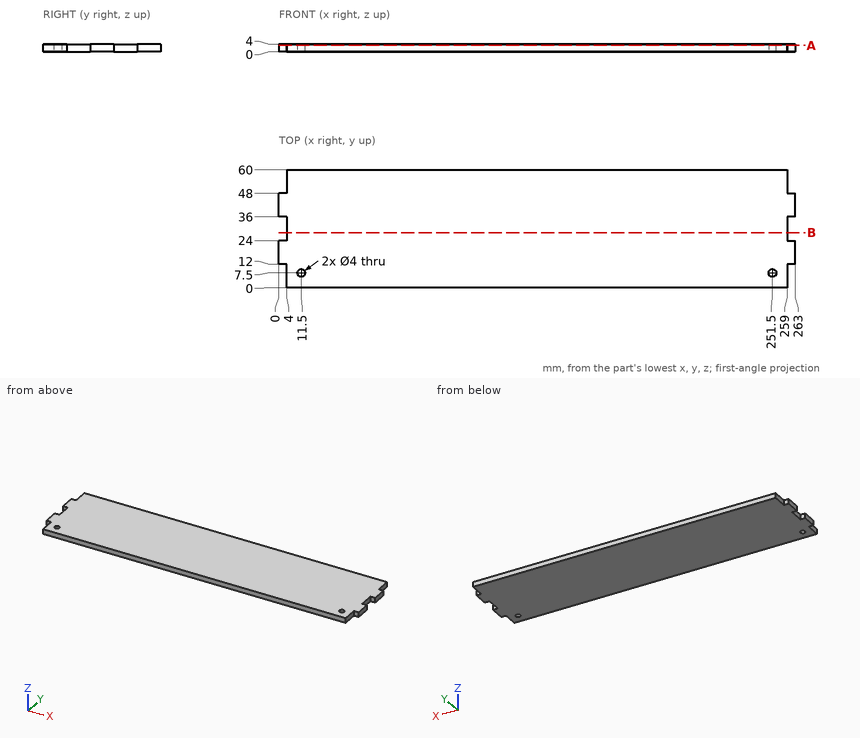
Study the drawing (mm; zero at the part's minimum x, y, z) and answer. Round coordinates to 2 decimals unless told otherwise and drop trailing zeros. Loops run counter-clockwise (first coordinate to the right, second up) from the corner with the lowest first, then second, coordinate; pieces in that order, holes last. Notation, with made-up numbers: (-1.5, 47.25) -> (7.5, 47.25) arc R18 ccw to (7.5, 59.25) -> close; hole circle Ø4 at (-26.5, 55.25). An arc over 180 degrees is marked (long way). One line per item, written item: value.
1) A cutting plane is placed at B-B (y = 28). Determine the outline of the cut face in (x, z), and give its area (3 significant figures).
Answer list:
outline: (4, 0) -> (259, 0) -> (259, 4) -> (4, 4) -> close
area: 1,020 mm²
2) Flat-ended cylindrical pins translate along their axes: P1, Ø1.2, axis at x = 2, z = 1, coming from the -Y side; P2, Ø1.2, axis at x = 2, z = 1, coming from the +Y side; P3, Ø1.2, axis at y = 31.5, z = 2, coming from the -X side. Find the tip coordinate at first contact, or state that the pin passes through.
Answer list:
P1: stops at y = 12
P2: stops at y = 48
P3: stops at x = 4
3) Consider L1, parallel to X at y = 7.5, z = 1.95; L2, parallel to Y at x = 251.5, z = 2.1; L3, parallel to X at y = 54.5, z = 2.5. Determine where each line is inside the solid, lowest interval first. Write a range as [from, to].
Answer list:
L1: x = [4, 9.5], [13.5, 249.5], [253.5, 259]
L2: y = [0, 5.5], [9.5, 60]
L3: x = [4, 259]
4) A cutting plane is placed at A-A (z = 3.3). Determine the outline of the cut face in (x, y).
Answer list:
outline: (0, 12) -> (4, 12) -> (4, 0) -> (259, 0) -> (259, 12) -> (263, 12) -> (263, 24) -> (259, 24) -> (259, 36) -> (263, 36) -> (263, 48) -> (259, 48) -> (259, 60) -> (4, 60) -> (4, 48) -> (0, 48) -> (0, 36) -> (4, 36) -> (4, 24) -> (0, 24) -> close; hole circle Ø4 at (11.5, 7.5); hole circle Ø4 at (251.5, 7.5)
